Autodesk Inventor part; units mm, degrees
ref_plane "YZ Plane" through (0, 0, 0) normal (1, 0, 0) x (0, 1, 0)
ref_plane "XZ Plane" through (0, 0, 0) normal (0, 1, 0) x (-1, 0, 0)
ref_plane "XY Plane" through (0, 0, 0) normal (0, 0, 1) x (1, 0, 0)
sketch "Sketch1" plane through (0, 0, 0) normal (0, 0, 1) x (1, 0, 0)
  arc A0 (5.9638, 43.7198) -> (6.8764, 42.8382) centre (5.7537, 42.5892) ccw
  arc A1 (6.2105, 45.0471) -> (8.2537, 42.5823) centre (5.7537, 42.5892) ccw
  arc A2 (19.5035, 33.7876) -> (21.3811, 31.3432) centre (18.8812, 31.3663) ccw
  line L0 (6.2105, 45.0471) -> (9.4943, 44.4368)
  line L1 (9.4943, 44.4368) -> (21.4548, 39.3429)
  line L2 (21.4548, 39.3429) -> (21.3811, 31.3432)
  line L3 (5.9638, 43.7198) -> (9.3282, 43.0946)
  line L4 (9.3282, 43.0946) -> (20.2464, 38.4445)
  line L5 (20.2464, 38.4445) -> (20.1811, 31.3543)
  line L6 (6.8764, 42.8382) -> (8.2537, 42.5823)
  line L7 (19.5035, 33.7876) -> (19.4918, 32.5139)
  arc A3 (19.4918, 32.5139) -> (20.1811, 31.3543) centre (18.8812, 31.3663) ccw
  line L8 (5.7537, 42.5892) -> (18.8812, 31.3663) construction
  circle A4 centre (5.7537, 42.5892) radius 1.2
  point P0 (0, 0)
  dimension "d0" = 5
  dimension "d1" = 5
  dimension "d2" = 1.3
  dimension "d5" = 1.35
  dimension "d8" = 8
  dimension "d9" = 0.7
  dimension "d10" = 0.7
  dimension "d12" = 1.2
  dimension "d18" = 2.3
  dimension "d19" = 30
  dimension "d20" = 13
  dimension "d21" = 50
extrude "Extrusion1" add sketch "Sketch1" along normal mid plane 10 contours A0 L6 A4 L3 | A4 L6 A1 L0 L1 L2 A2 L7 A3 L5 L4 L3 picked at (6.096, 43.7118)
fillet "Fillet1" radius 2 2 edges at (20.2464, 38.4445, 0) (9.3282, 43.0946, 0)
fillet "Fillet1" radius 3 2 edges at (9.4943, 44.4368, 0) (21.4548, 39.3429, 0)
properties part number "Linkage for full overlay hinge" material "Steel"
Can you work these out from the model? Positions are in its coordinate system, mm. A direction names the side the tool comes from. Coordinates: 2 decimals unless noted, no trailing zeros. Order: outer loops, then holes, each group sorted by start corner. A loop starts at its lowest first (then second) coordinate and runs counter-clockwise, first axis right, second up.
1. If we section it at D-D (x = 13.75): Please give me the cut outline in (y, z).
2. I need wall thicknesses on line 1 (Y direction, x = 18.5, z = -3.5); line 2 (X direction, y = 41.75, z = -0.25); line 3 (Y direction, x = 18.25, z = 1.5). Which ranges of each line are inside material? Lowest first, please.
3. For faces 4 (the face through (7.56, 42.71, -0.07)), 5 (the face through (7.67, 44.776, -0.07)), 6 (the face through (19.917, 38.209, 0.07)), which set-ups out of +Z, -Z, +X, -X, +Y, -Y let a thin tool reach every point of the face, with its end or its side?
4. If we section it at C-C (y = 30.5): Please give me the cut outline in (x, z).
5. If we section it at B-B (z = 2.5): Please give me the cut outline in (x, y), then the cut area to 3 significant figures.
6. If we section it at A-A (y = 43.5): Please give me the cut outline in (x, z), then the cut area to 3 significant figures.
7. Thinking about a two-plate mould opening in X: for faces 1 (the face through (14.636, 42.247, -0.07)), 2 (the face through (4.985, 41.734, -0.07)), 3 (the face through (14.3, 41.2, 5)), which applies, +X half, -X half, draft (parallel to the pull), parting line (faces both ways), or undercut?
8. I'm going to push flat-ended pins straight in: pin 1 (3 mm diameter, centred on y = 38, z = -0.5, fed in from -X); pin 2 (2.5 mm diameter, centred on x = 18.88, y = 31.37, fed in from -Z); pin 3 (1.5 mm diameter, centred on x = 17.5, z = 2.5, fed in from +Y); pin 4 (3 mm diameter, centred on x = 13, z = 2, fed in from -Y). Where does each tip first touch, or does it pass through?
Entries:
1. outline: (41.21, -5) - (42.62, -5) - (42.62, 5) - (41.21, 5) - close
2. line 1: y = 28.9 to 30.12, 32.61 to 33.84, 39.19 to 40.6
2. line 2: x = 3.4 to 4.97, 6.54 to 8.11, 12.49 to 15.8
2. line 3: y = 28.95 to 30.23, 32.5 to 33.79, 39.29 to 40.71
3. face 4: +Z, -Z
3. face 5: +Z, -Z, +X, +Y
3. face 6: +Z, -Z, -X
4. outline: (16.54, -5) - (17.91, -5) - (17.91, 5) - (16.54, 5) - close; (19.85, -5) - (21.23, -5) - (21.23, 5) - (19.85, 5) - close
5. outline: (5.96, 43.72) - (9.11, 43.13) arc R2 cw to (9.53, 43.01) - (19.02, 38.97) arc R2 cw to (20.23, 37.11) - (20.18, 31.35) arc R1.3 cw (long way) to (19.49, 32.51) - (19.5, 33.79) arc R2.5 ccw (long way) to (21.38, 31.34) - (21.44, 37.34) arc R3 ccw to (19.61, 40.13) - (9.8, 44.31) arc R3 ccw to (9.17, 44.5) - (6.21, 45.05) arc R2.5 ccw (long way) to (8.25, 42.58) - (6.88, 42.84) arc R1.15 cw (long way) to start
5. area: 53.1 mm2
6. outline: (3.43, -5) - (5.05, -5) - (5.05, 5) - (3.43, 5) - close; (7.15, -5) - (11.69, -5) - (11.69, 5) - (7.15, 5) - close
6. area: 61.7 mm2
7. face 1: +X half
7. face 2: undercut
7. face 3: draft
8. pin 1: stops at x = 17.77
8. pin 2: passes through
8. pin 3: stops at y = 41.35
8. pin 4: stops at y = 40.89
